Input: part model. Units: mm. Frame: model coordinates. A direction names the side the tool comes from. Round coordinates to 2 decimals unless told otherwise and drop trailing zeros. Order: outer loops, then holes, each group sorted by start corner. A loop starts at its lowest first (then second) coordinate and runs counter-clockwise, first axis right, second up.
Item 1: Cut plane D-D on z = -16.25. Output: boundary loops of the cut face in (x, y).
Item 2: Line query: L1, parallel to Z at x = 36, y = 3.5; L2, parallel to X at y = 1.8, z = -11.5; L3, parallel to Z at x = -66, y = 2.2. Output: solid intervals per line, ascending.
Item 3: First-contact query: pin 1 (2.5 mm diameter, centred on x = -10, y = 2, fed in from -Z); pin 2 (11.5 mm diameter, centred on x = 83.77, z = -8.04, fed in from -Y); pin 3 (3.5 mm diameter, centred on x = -4.23, z = -8.04, fed in from +Y); pin 4 (2.5 mm diameter, centred on x = -5.5, y = 3.5, fed in from +Z). Flat tips, straight axial feed; report the tip coordinate or a pass-through.
Item 4: Cut plane A-A on z = -7.75. Output: boundary loops of the cut face in (x, y).
Item 5: Reachability of faces 1 (the flat face through (3, 2, -19.038)), 2 (the cylindrical face through (73.37, 2.465, 3.226)) from +Z, -Z, +X, -X, +Y, -Y: full face, straight path, thin tool, end or side. Return the list, or none.
Item 6: Cut plane C-C on x = 58. Output: boundary loops of the cut face in (y, z), then the cut area to 3 significant figures.
Item 7: Mould query, pull axis Z, two halves, no side actions, for faces 3 (the cylindrical face through (-59.77, 2.46, -8.62)), 4 (the flat face through (5, 2, 2.962)), 5 (the cylindrical face through (73.33, 2.46, -19.29)). Classes: released by +Z, released by -Z, zero draft, split by the parting line, or undercut.
Item 8: Cut plane B-B on y = 3. Output: boundary loops of the cut face in (x, z), then the cut area to 3 significant figures.
```python
from build123d import *

# Parameters (mm, degrees)
SKETCH_1_R      = 4.5
SKETCH_1_R_2    = 2
EXTRUDE_1_DEPTH = 5


with BuildPart() as part:
    # 草图1 → 凸台-拉伸1 (new body)
    with BuildSketch(Plane(origin=(0, 0, 0), x_dir=(1, 0, 0), z_dir=(0, 1, 0))):
        with BuildLine():
            Line((-64.232662192, 19.03803132), (71.767337808, 19.03803132))
            ThreePointArc((71.767337808, 19.03803132), (73.348476638, 19.29461483), (74.767337808, 20.03803132))
            ThreePointArc((74.767337808, 20.03803132), (98.767337808, 8.03803132), (74.767337808, -3.96196868))
            ThreePointArc((74.767337808, -3.96196868), (73.348476638, -3.21855219), (71.767337808, -2.96196868))
            Line((71.767337808, -2.96196868), (-64.232662192, -2.96196868))
            ThreePointArc((-64.232662192, -2.96196868), (-75.232662192, 8.03803132), (-64.232662192, 19.03803132))
        make_face()
        with Locations(Location((-64.232662192, 8.03803132, 0), (0, 0, 270))):
            Circle(SKETCH_1_R, mode=Mode.SUBTRACT)
        with Locations(Location((83.767337808, 8.03803132, 0), (0, 0, 270))):
            Circle(SKETCH_1_R, mode=Mode.SUBTRACT)
        with Locations(Location((-4.232662192, 8.03803132, 0), (0, 0, 270))):
            Circle(SKETCH_1_R_2, mode=Mode.SUBTRACT)
        with Locations(Location((23.767337808, 8.03803132, 0), (0, 0, 270))):
            Circle(SKETCH_1_R_2, mode=Mode.SUBTRACT)
    extrude(amount=EXTRUDE_1_DEPTH)


solid = part.part
```
From the geometry:
1. outline: (-71.55, 0) - (96.32, 0) - (96.32, 5) - (-71.55, 5) - close
2. L1: z = -19.04 to 2.96
2. L2: x = -74.67 to -67.11, -61.36 to 80.89, 86.64 to 98.36
2. L3: z = -18.9 to -12.18, -3.9 to 2.82
3. pin 1: stops at z = -19.04
3. pin 2: stops at y = 0
3. pin 3: passes through
3. pin 4: stops at z = 2.96
4. outline: (-75.23, 0) - (-68.72, 0) - (-68.72, 5) - (-75.23, 5) - close; (-59.74, 0) - (-6.21, 0) - (-6.21, 5) - (-59.74, 5) - close; (-2.25, 0) - (21.79, 0) - (21.79, 5) - (-2.25, 5) - close; (25.75, 0) - (79.28, 0) - (79.28, 5) - (25.75, 5) - close; (88.26, 0) - (98.76, 0) - (98.76, 5) - (88.26, 5) - close
5. face 1: -Z, -X, +Y, -Y
5. face 2: +Z, -X, +Y, -Y
6. outline: (0, -19.04) - (5, -19.04) - (5, 2.96) - (0, 2.96) - close
6. area: 110 mm2
7. face 3: undercut
7. face 4: released by +Z
7. face 5: released by -Z
8. outline: (-64.23, -19.04) - (71.77, -19.04) arc R5 cw to (74.77, -20.04) arc R15 ccw (long way) to (74.77, 3.96) arc R5 cw to (71.77, 2.96) - (-64.23, 2.96) arc R11 ccw to start; hole circle Ø9 at (-64.23, -8.04); hole circle Ø4 at (-4.23, -8.04); hole circle Ø4 at (23.77, -8.04); hole circle Ø9 at (83.77, -8.04)
8. area: 3,700 mm2
